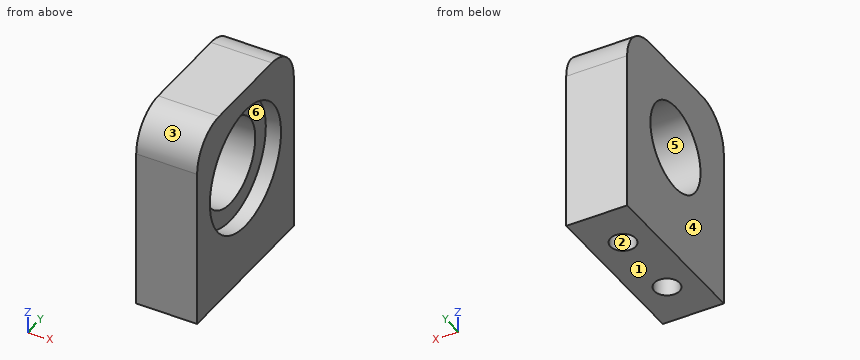
from build123d import *

# Parameters (mm, degrees)
SKETCH1_W                      = 26
SKETCH1_H                      = 22
BOSS_EXTRUDE1_DEPTH            = 8
SKETCH2_R                      = 8.1
CUT_EXTRUDE1_DEPTH             = 2
F_3_3_3_3_DIAMETER_HOLE1_D     = 3.3
F_3_3_3_3_DIAMETER_HOLE1_DEPTH = 6
F_3_3_3_3_DIAMETER_HOLE1_TIP   = 0.991420021
M10_CLEARANCE_HOLE1_D          = 11.4
FILLET1_R                      = 5


with BuildPart() as part:
    # Sketch1 → Boss-Extrude1 (new body)
    with BuildSketch(Plane(origin=(8, 0, 0), x_dir=(0, 0, -1), z_dir=(1, 0, 0))):
        with Locations((-9, 11)):
            Rectangle(SKETCH1_W, SKETCH1_H)
    extrude(amount=-BOSS_EXTRUDE1_DEPTH)

    # Sketch2 → Cut-Extrude1 (cut)
    with BuildSketch(Plane(origin=(8, 0, 0), x_dir=(0, 0, -1), z_dir=(1, 0, 0))):
        with Locations((-11, 11)):
            Circle(SKETCH2_R)
    extrude(amount=-CUT_EXTRUDE1_DEPTH, mode=Mode.SUBTRACT)

    # Ø3.3 (3.3) Diameter Hole1
    with Locations(Plane(origin=(0, 0, -4), x_dir=(-1, 0, 0), z_dir=(0, 0, -1))):
        with Locations((-4, 16), (-4, 6)):
            Hole(F_3_3_3_3_DIAMETER_HOLE1_D / 2, depth=F_3_3_3_3_DIAMETER_HOLE1_DEPTH)
            with Locations((0, 0, -(F_3_3_3_3_DIAMETER_HOLE1_DEPTH + F_3_3_3_3_DIAMETER_HOLE1_TIP / 2))):  # 118° drill point
                Cone(0, F_3_3_3_3_DIAMETER_HOLE1_D / 2, F_3_3_3_3_DIAMETER_HOLE1_TIP, mode=Mode.SUBTRACT)

    # M10 Clearance Hole1 (through all)
    with Locations(Plane(origin=(6, 0, 0), x_dir=(0, 0, -1), z_dir=(1, 0, 0))):
        with Locations((-11, 11)):
            Hole(M10_CLEARANCE_HOLE1_D / 2)

    # Fillet1
    fillet1_edges = [part.edges().sort_by_distance(p)[0] for p in [
        (4, 0, 22),
        (4, 22, 22),
    ]]
    fillet(fillet1_edges, radius=FILLET1_R)


solid = part.part
The listing builds one solid part. Answer for the finished solid, in the listing's coordinates (mm). Face numbers are marked on the shaded views. A direction names the side the tool comes from. Coordinates: 2 decimals unless noted, no trailing zeros. Write each loop counter-clockwise with the first axis right and the second up, starting at its lowest first coordinate (ties: lowest second). Pieces come first, ordered by that corner, then holes. Notation, with made-up numbers: (77.25, 34) -> (120.25, 34) arc R26 ccw to (120.25, 60) -> close; hole circle Ø10 at (7.5, 65.5). An arc over 180 degrees is marked (long way). One line per question, with ' | ' between items.
1. Section D-D (y = 18) is taken. Determine the outline of the cut face in (x, z).
Verdict:
outline: (0, -4) -> (8, -4) -> (8, 6.92) -> (6, 6.92) -> (6, 15.08) -> (8, 15.08) -> (8, 21.9) -> (0, 21.9) -> close
2. Section A-A (z = 11) is taken. Determine the outline of the cut face in (x, y).
Verdict:
outline: (0, 0) -> (8, 0) -> (8, 2.9) -> (6, 2.9) -> (6, 5.3) -> (0, 5.3) -> close; (0, 16.7) -> (6, 16.7) -> (6, 19.1) -> (8, 19.1) -> (8, 22) -> (0, 22) -> close
3. Straight lines are drawn through the part: line 1 (Y direction, x = 4, z = -1.85); line 2 (Y direction, x = 6.9, z = 11); line 3 (Y direction, x = 1.9, z = 11). For each, find the intervals that lie inside material, in ascending order.
Verdict:
line 1: y = 0 to 4.35, 7.65 to 14.35, 17.65 to 22 | line 2: y = 0 to 2.9, 19.1 to 22 | line 3: y = 0 to 5.3, 16.7 to 22
4. Section B-B (y = 11) is taken. Determine the outline of the cut face in (x, z), and give its area (3 significant figures).
Verdict:
outline: (0, -4) -> (8, -4) -> (8, 2.9) -> (6, 2.9) -> (6, 5.3) -> (0, 5.3) -> close; (0, 16.7) -> (6, 16.7) -> (6, 19.1) -> (8, 19.1) -> (8, 22) -> (0, 22) -> close | area: 107 mm^2
5. Given pin 1 Ø9.5 at (y, z) = (11, 11) entering from +X; pin 2 Ø4 at (x, y) = (3, 2.5) entering from +Z; pin 3 Ø2 at (x, y) = (4, 16) entering from -Z, each flat-ended and moving along its own axis, determine where each tip first touches the part or whether it passes through.
Verdict:
pin 1: passes through | pin 2: stops at z = 21.97 | pin 3: stops at z = 2.39
6. Section C-C (z = 1) is taken. Determine the outline of the cut face in (x, y), and give its area (3 significant figures).
Verdict:
outline: (0, 0) -> (8, 0) -> (8, 22) -> (0, 22) -> close; hole circle Ø3.3 at (4, 6); hole circle Ø3.3 at (4, 16) | area: 159 mm^2
7. For a pull along Z with two mould halves and no side action, classify the marked faces 3, 4, 5 and 6 as released by +Z, released by -Z, zero draft, split by the parting line, or undercut.
Verdict:
face 3: released by +Z | face 4: zero draft | face 5: undercut | face 6: undercut
8. Which of the six approach directions +Z, -Z, +X, -X, +Y, -Y give full straight-line access (tool end or side, diameter ignored) to the marked faces 1 and 2?
Verdict:
face 1: -Z, +X, -X, +Y, -Y | face 2: -Z
